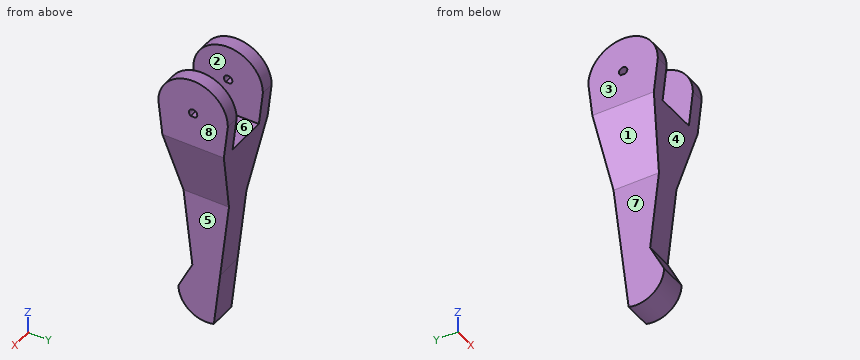
from build123d import *

# Parameters (mm, degrees)
BOSS_EXTRUDE1_DEPTH     = 50
CUT_EXTRUDE1_DEPTH      = 179.955301682
CUT_EXTRUDE1_DEPTH_BACK = 179.955301682
CUT_EXTRUDE5_DEPTH      = 179.955301682
CUT_EXTRUDE5_DEPTH_BACK = 179.955301682
SKETCH5_W               = 30
SKETCH5_H               = 50
CUT_EXTRUDE6_DEPTH      = 176.356779168
CUT_EXTRUDE6_DEPTH_BACK = 176.356779168
CUT_EXTRUDE7_DEPTH      = 179.955301682
CUT_EXTRUDE7_DEPTH_BACK = 179.955301682


with BuildPart() as part:
    # Sketch1 → Boss-Extrude1 (new body)
    with BuildSketch(Plane(origin=(0, 0, 0), x_dir=(0, 0, -1), z_dir=(1, 0, 0))):
        with BuildLine():
            Line((0, 25), (130, 10))
            Line((130, 10), (150, 20))
            ThreePointArc((150, 20), (170, 0), (150, -20))
            Line((150, -20), (130, -10))
            Line((130, -10), (0, -25))
            ThreePointArc((0, -25), (-25, 0), (0, 25))
        make_face()
    extrude(amount=BOSS_EXTRUDE1_DEPTH)

    # Sketch3 → Cut-Extrude1 (cut, two sides: drawn at the far end of the back side and taken through both)
    with BuildSketch(Plane(origin=(0, 0, 0), x_dir=(1, 0, 0), z_dir=(0, 1, 0)).offset(-CUT_EXTRUDE1_DEPTH_BACK)):
        Polygon((15, 170), (15, 75), (0, 25), (-45.149252574, 25), (-45.149252574, 231.988814071), (97.66148476, 231.988814071), (97.66148476, 25), (50, 25), (35, 75), (35, 170), align=None)
    extrude(amount=CUT_EXTRUDE1_DEPTH + CUT_EXTRUDE1_DEPTH_BACK, mode=Mode.SUBTRACT)

    # Sketch5 → Cut-Extrude5 (cut, two sides: drawn at the far end of the back side and taken through both)
    with BuildSketch(Plane(origin=(0, 0, 0), x_dir=(1, 0, 0), z_dir=(0, 1, 0)).offset(-CUT_EXTRUDE5_DEPTH_BACK)):
        with Locations((25, 0)):
            Rectangle(SKETCH5_W, SKETCH5_H)
    extrude(amount=CUT_EXTRUDE5_DEPTH + CUT_EXTRUDE5_DEPTH_BACK, mode=Mode.SUBTRACT)

    # Sketch6 → Cut-Extrude6 (cut, two sides: drawn at the far end of the back side and taken through both)
    with BuildSketch(Plane.ZY.offset(-15).offset(-CUT_EXTRUDE6_DEPTH_BACK)):
        Polygon((-130, 10), (-189.136006784, 3.176614602), (-191.554152375, 31.687839347), (-130.171893451, 25.24666108), align=None)
    extrude(amount=CUT_EXTRUDE6_DEPTH + CUT_EXTRUDE6_DEPTH_BACK, mode=Mode.SUBTRACT)

    # Sketch7 → Cut-Extrude7 (cut, two sides: drawn at the far end of the back side and taken through both)
    with BuildSketch(Plane.ZY.offset(-CUT_EXTRUDE7_DEPTH_BACK)):
        with BuildLine():
            Line((-2.5, 1.658312395), (-2.5, -1.658312395))
            ThreePointArc((-2.5, -1.658312395), (3, 0), (-2.5, 1.658312395))
        make_face()
    extrude(amount=CUT_EXTRUDE7_DEPTH + CUT_EXTRUDE7_DEPTH_BACK, mode=Mode.SUBTRACT)


solid = part.part
CAD build for the part. Positions are in the model's coordinates, mm. Face numbers are marked on the shaded views. A direction names the side the tool comes from. Round coordinates to 2 decimals unless told otherwise and drop trailing zeros. Order: outer loops, then holes, each group sorted by start corner. A loop starts at its lowest first (then second) coordinate and runs counter-clockwise, first axis right, second up. Notation, with made-up numbers: (-26, 41.25) - (-22, 41.25) arc R22 cw to (-22, 66.25) - close; hole circle Ø2 at (53, 17.5). An arc over 180 degrees is marked (long way). Return JSON: item names as keys, results as strings.
(1) Tool access for the marked faces 1, 2, 3, 4 and 5: list every direction of +Z, -Z, +X, -X, +Y, -Y with a clear straight run to the whole face (end or side of a thin tool).
Answer key:
{"face 1": "-Z, -X, +Y, -Y", "face 2": "+Z, +Y, -Y", "face 3": "+Z, -Z, -X, +Y, -Y", "face 4": "+X, -X, -Y", "face 5": "-Z, +X, +Y, -Y"}
(2) Pin check, flat tips, straight feed: pin 1 Ø2.5 at (x, y) = (7, 0.5) entering from +Z; pin 2 Ø10 at (x, z) = (15, -141.5) entering from +Y; pin 3 Ø3 at (x, y) = (41.5, -18.5) entering from +Z. Stop position of each tip, or through.
Answer key:
{"pin 1": "stops at z = 25", "pin 2": "stops at y = 9.25", "pin 3": "stops at z = 18.33"}
(3) Cut at B-B (z = -71.5). Give the cut face in (x, y), then the cut area to 3 significant figures.
Answer key:
{"outline": "(13.95, -16.75) - (36.05, -16.75) - (36.05, 16.75) - (13.95, 16.75) - close", "area": "740 mm^2"}
(4) Pull direction X, two halves, no side cores. Call the marked faces 6, 7 and 8: +X half, -X half, draft (parallel to the pull), parting line (faces both ways), or undercut.
Answer key:
{"face 6": "undercut", "face 7": "-X half", "face 8": "+X half"}
(5) Cut at C-C (z = -113). Give the cut face in (x, y).
Answer key:
{"outline": "(15, -11.96) - (35, -11.96) - (35, 11.96) - (15, 11.96) - close"}
(6) Cut at A-A (y = 8). Give the cut face in (x, z), then the cut area to 3 significant figures.
Answer key:
{"outline": "(0, -25) - (15, -75) - (15, -147.33) - (35, -147.33) - (35, -75) - (50, -25) - (50, 23.69) - (40, 23.69) - (40, -25) - (10, -25) - (10, 23.69) - (0, 23.69) - close", "area": "4,170 mm^2"}
(7) Wall check: probe 1 along X at (y, z) = (5, 3); probe 2 along X at (y, z) = (8.5, -90.5); probe 3 along Y at (x, z) = (32, -135). Give the ranges that are in metal, low to high. Write a range as from..to.
Answer key:
{"probe 1": "x = 0..10, 40..50", "probe 2": "x = 15..35", "probe 3": "y = -12.5..9.42"}
